from build123d import *

# Parameters (mm, degrees)
CHAMFER2_SIZE = 6
CHAMFER3_SIZE = 3
CHAMFER4_SIZE = 1
FILLET1_R     = 6
CHAMFER5_SIZE = 1


with BuildPart() as part:
    # Sketch1 → Revolve2 (revolve)
    with BuildSketch(Plane.XY, mode=Mode.PRIVATE) as revolve2_sk:
        Polygon((0, -10), (0, -20), (50, -20), (50, -13), (52, -13), (52, -14), (90, -14), (90, -8), (150, -8), (150, -4), (125, -4), (125, 0), (36, 0), (36, -10), align=None)
    revolve(revolve2_sk.sketch.rotate(Axis((0, 0, 0), (1, 0, 0)), 270), axis=Axis((0, 0, 0), (1, 0, 0)))

    # Chamfer2
    chamfer2_edges = [part.edges().sort_by_distance(p)[0] for p in [
        (0, 0, -20),
        (50, 0, -20),
    ]]
    chamfer(chamfer2_edges, length=CHAMFER2_SIZE)

    # Chamfer3
    chamfer3_edges = [part.edges().sort_by_distance(p)[0] for p in [
        (0, 0, -10),
    ]]
    chamfer(chamfer3_edges, length=CHAMFER3_SIZE)

    # Chamfer4
    chamfer4_edges = [part.edges().sort_by_distance(p)[0] for p in [
        (150, 0, -4),
    ]]
    chamfer(chamfer4_edges, length=CHAMFER4_SIZE)

    # Fillet1
    fillet1_edges = [part.edges().sort_by_distance(p)[0] for p in [
        (90, 0, -8),
    ]]
    fillet(fillet1_edges, radius=FILLET1_R - 0.0001)  # a hair under: the kernel refuses the full size

    # Chamfer5
    chamfer5_edges = [part.edges().sort_by_distance(p)[0] for p in [
        (52, 0, -14),
    ]]
    chamfer(chamfer5_edges, length=CHAMFER5_SIZE - 0.0001)  # a hair under: the kernel refuses the full size


solid = part.part
The model under review builds one solid part; all positions refer to its coordinate system, in mm. A direction names the side the tool comes from. Give positions to 0.01 mm unless a question says otherwise; leave off trailing zeros. Loops run counter-clockwise (first coordinate to the right, second up) from the corner with the lowest first, then second, coordinate; pieces in that order, holes last. Notation, with made-up numbers: (-1, 30) -> (40, 30) arc R6 ccw to (40, 36) -> close; hole circle Ø8 at (-18, 13.25). An arc over 180 degrees is marked (long way). Write each question's results on one line, items separated by ' | '.
1) For line 1 along Y through (x, z) = (15, 0); line 2 along Y through (x, z) = (130.25, 0); line 3 along Z through (x, y) = (84.5, -0.5), list the stretches that pass through material, from the lowest coordinate up. Write a range as from..to.
Conclusion:
line 1: y = -20..-10, 10..20 | line 2: y = -8..-4, 4..8 | line 3: z = -13.99..13.99
2) Tool access review of faces 5 (the face through (123.38, 7.81, -1.73)), 6 (the face through (19.27, 9.76, -2.17)), 7 (the face through (51.014, 7.91, -10.316)): name each direction out of +Z, -Z, +X, -X, +Y, -Y from which nothing blocks a thin tool from reaching the whole face with its end or side.
Conclusion:
face 5: +X | face 6: -X | face 7: none
3) Draft analysis for pull direction Y (two halves, no side actions). For faces 1 (the face through (36, 0, 0)), 2 (the face through (49.71, 13.95, -3.1)), 3 (the face through (136.832, 3.905, -0.867)), 4 (the face through (50, 9.3, 9.3)), state which applies: pulls with the +Y half, pulls with the -Y half, needs draft (parallel to the pull), parting line crosses it, or undercut.
Conclusion:
face 1: undercut | face 2: parting line crosses it | face 3: undercut | face 4: needs draft
4) Take a section at A-A, the plane x = 109. Give the boundary of the cut face in (y, z).
Conclusion:
outline: circle Ø16 at (0, 0)
5) Insertion check: pin 1 Ø16 at (y, z) = (0, 0) entering from -X; pin 2 Ø2 at (x, z) = (15, -15.5) entering from -Y (3 decimals); pin 3 Ø1.5 at (y, z) = (12.5, -10) entering from +X. Each pin has a flat end and moves straight along its axis. Give the tip position at first contact, or say it passes through.
Conclusion:
pin 1: stops at x = 36 | pin 2: stops at y = -13.775 | pin 3: stops at x = 48.74
